Autodesk Inventor part; units mm, degrees
ref_plane "YZ Plane" through (0, 0, 0) normal (1, 0, 0) x (0, 1, 0)
ref_plane "XZ Plane" through (0, 0, 0) normal (0, 1, 0) x (-1, 0, 0)
ref_plane "XY Plane" through (0, 0, 0) normal (0, 0, 1) x (1, 0, 0)
sketch "Sketch1" plane through (0, 0, 0) normal (0, 0, 1) x (1, 0, 0)
  circle A0 centre (0, 0) radius 10
  dimension "d0" = 20
extrude "Extrusion1" add sketch "Sketch1" along normal blind 18
sketch "Sketch2" plane through (0, 0, 18) normal (0, 0, 1) x (1, 0, 0)
  line L0 (0, 0) -> (0, 4) construction
  line L1 (0, 4) -> (-9.1652, 4)
  circle A0 centre (0, 0) radius 10
  line L2 (0, 4) -> (9.1652, 4)
  line L3 (0, 0) -> (0, -4) construction
  line L4 (0, -4) -> (9.1652, -4)
  line L5 (0, -4) -> (-6.1702, -4)
  point P0 (-8, -6)
  dimension "d3" = 4
  dimension "d4" = 4
extrude "Extrusion2" cut sketch "Sketch2" against normal blind 4
sketch "Sketch3" plane through (0, 0, 0) normal (0, 0, -1) x (-1, 0, 0)
  circle A0 centre (0, 0) radius 3
  dimension "d7" = 6
extrude "Extrusion3" cut sketch "Sketch3" against normal blind 10
thread "Thread1"
sketch "Sketch7" plane through (0, 0, 14) normal (0, 0, 1) x (1, 0, 0)
  line L0 (0, 0) -> (0, -6) construction
  line L1 (0, -6) -> (-8, -6)
  circle A0 centre (0, 0) radius 10
  line L2 (0, -6) -> (8, -6)
  line L3 (8, 6) -> (-8, 6)
  dimension "d21" = 6
extrude "Extrusion5" add sketch "Sketch7" along normal blind 6 contours L2 A0 L1 | A0 L3
sketch "Sketch8" plane through (0, 0, 14) normal (0, 0, 1) x (1, 0, 0)
  circle A0 centre (0, 0) radius 4
  dimension "d24" = 8
extrude "Extrusion6" add sketch "Sketch8" along normal blind 15
thread "Thread4"
chamfer "Chamfer1" distance 5 angle 45 1 edges at (-10, 0, 0)
properties material "Aluminum 6061"
Check sheet for the modelled part. Datum: model origin and axes. Units: mm. A direction names the side the tool comes from. Round coordinates to 2 decimals unless told otherwise and drop trailing zeros. Write each loop counter-clockwise with the first axis right and the second up, starting at its lowest first coordinate (ties: lowest second). Pieces come first, ordered by that corner, then holes. Notation, with made-up numbers: (61, -29.75) -> (97, -29.75) arc R26 ccw to (97, -11.75) -> close; hole circle Ø2 at (62, 73.5). An arc over 180 degrees is marked (long way). Put each result on its own line as item: value.
(1) Mould release check, pull along X, two halves, no side actions. Record for faces 6 (the face through (-1.152, -5.186, 0.313)), 7 (the face through (0, 0, 10)), 8 (the face through (0, 0, 29)), 9 (the face through (3, 0, 5)): released by +X, released by -X, zero draft, split by the parting line, or undercut.
Values found:
face 6: split by the parting line
face 7: undercut
face 8: zero draft
face 9: undercut
(2) Sectioned sample at A-A (z = 15.25). Enter the section's corners in (x, y).
Values found:
outline: (-8, -6) arc R10 ccw to (8, -6) -> close; (-8, 6) -> (8, 6) arc R10 ccw to start; circle Ø8 at (0, 0)
(3) Go/stop test with flat-tipped pins: pin 1 Ø10 at (y, z) = (1.5, 26) entering from -X; pin 2 Ø2 at (x, y) = (3, -8.5) entering from +Z; pin 3 Ø6.5 at (x, z) = (2.5, 18) entering from -Y; pin 4 Ø5 at (x, z) = (4.5, 19) entering from +Y. Record where each tip stops, or that it passes through.
Values found:
pin 1: stops at x = -4
pin 2: stops at z = 20
pin 3: stops at y = -10
pin 4: stops at y = 9.8
(4) Sectioned sample at D-D (z = 8.75). Enter the section's corners in (x, y).
Values found:
outline: circle Ø20 at (0, 0); hole circle Ø6 at (0, 0)
(5) Sectioned sample at C-C (y = 0). Enter the section's corners in (x, z), plus the area to 3 significant figures.
Values found:
outline: (-10, 5) -> (-5, 0) -> (-3, 0) -> (-3, 10) -> (3, 10) -> (3, 0) -> (5, 0) -> (10, 5) -> (10, 14) -> (4, 14) -> (4, 29) -> (-4, 29) -> (-4, 14) -> (-10, 14) -> close
area: 315 mm^2
(6) Material ranges on line 1 (Y direction, x = 0, z = 8.25); line 2 (Y direction, x = -3, z = 19.25); line 3 (Z direction, x = 4.25, y = -2.25), recorded low to high.
Values found:
line 1: y = -10 to -3, 3 to 10
line 2: y = -9.54 to -6, -2.65 to 2.65, 6 to 9.54
line 3: z = 0 to 14
(7) Tool access check on faces 1 (the face through (0, -8, 20)), 2 (the face through (-10, 0, 12)), 3 (the face through (-5, 0, 14)), 4 (the face through (0, 8, 20)), 5 (the face through (0, -6, 17)). Record the directions out of +Z, -Z, +X, -X, +Y, -Y that give a thin tool (end or side, any length) a straight path to the whole face; none if there is none.
Values found:
face 1: +Z, +X, -X, -Y
face 2: +Z, -Z
face 3: +Z
face 4: +Z, +X, -X, +Y
face 5: +Z, +X, -X
(8) Sectioned sample at B-B (x = 0). Enter the section's corners in (y, z), plus the area to 3 significant figures.
Values found:
outline: (-10, 5) -> (-5, 0) -> (-3, 0) -> (-3, 10) -> (3, 10) -> (3, 0) -> (5, 0) -> (10, 5) -> (10, 20) -> (6, 20) -> (6, 14) -> (4, 14) -> (4, 29) -> (-4, 29) -> (-4, 14) -> (-6, 14) -> (-6, 20) -> (-10, 20) -> close
area: 363 mm^2
